```python
from build123d import *

# Parameters (mm, degrees)
F0_R     = 6
F1_DEPTH = 25
F3_DEPTH = 12.5


with BuildPart() as f1:
    # F0 (on Front) → F1 (new body)
    with BuildSketch(Plane.XZ):
        with BuildLine():
            ThreePointArc((-34.439272, -8.041347), (-32.264663, -4.27924), (-31.509368, 0))
            ThreePointArc((-31.509368, 0), (-32.24635, 4.228641), (-34.370393, 7.958653))
            ThreePointArc((-34.370393, 7.958653), (-56.509252, 0.053811), (-34.439272, -8.041347))
        make_face()
        with Locations((-44.009368, 0)):
            Circle(F0_R, mode=Mode.SUBTRACT)
        with BuildLine():
            ThreePointArc((-34.370393, 7.958653), (-32.24635, 4.228641), (-31.509368, 0))
            ThreePointArc((-31.509368, 0), (-32.264663, -4.27924), (-34.439272, -8.041347))
            Line((-34.439272, -8.041347), (35.046161, -8.041347))
            ThreePointArc((35.046161, -8.041347), (30.99087, -0.068914), (34.935895, 7.958653))
            Line((34.935895, 7.958653), (-34.370393, 7.958653))
        make_face()
        with BuildLine():
            ThreePointArc((50.990632, 0), (45.432064, 8.959558), (34.935895, 7.958653))
            ThreePointArc((34.935895, 7.958653), (30.99087, -0.068914), (35.046161, -8.041347))
            ThreePointArc((35.046161, -8.041347), (45.493703, -8.928738), (50.990632, 0))
        make_face()
        with Locations((40.990632, 0)):
            Circle(F0_R, mode=Mode.SUBTRACT)
    extrude(amount=F1_DEPTH)

    # F2 (on Top) → F3 (intersect, symmetric)
    with BuildSketch(Plane.XY):
        Polygon((-27.554982, -9), (-56.499865, -9), (-56.499865, -18), (-26.767584, -18), (24.273953, -9), (51.126346, -9), (51.126346, 0), (23.486555, 0), align=None)
    extrude(amount=F3_DEPTH, both=True, mode=Mode.INTERSECT)


solid = f1.part
```
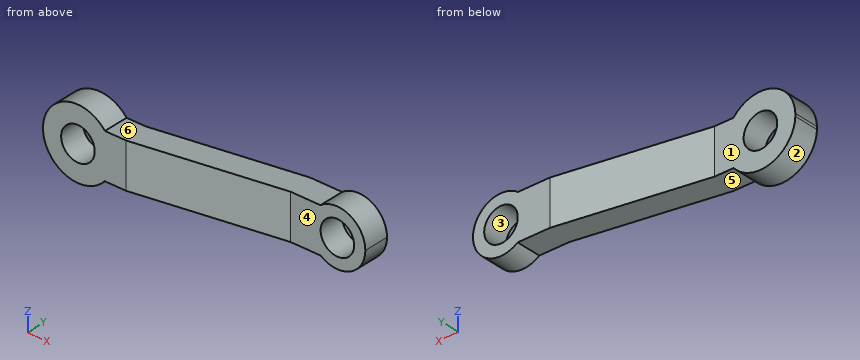
Can you work these out from the model? Positions are in its coordinate system, mm. Face numbers are marked on the shaded views. A direction names the side the tool comes from. Give positions to 0.01 mm unless a question says otherwise; leave off trailing zeros. Loops run counter-clockwise (first coordinate to the right, second up) from the corner with the lowest first, then second, coordinate; pieces in that order, holes last. Notation, with made-up numbers: M -28,-35 L -18,-35 A21 ccw -18,-9 Z; hole C -31.75,39.25 d3. An arc over 180 degrees is marked long. One line per item, written item: value.
(1) Will these pins go through, and if not, where does the flat tip stop? pin 1 (3 mm diameter, centred on x = -19.5, z = -6, fed in from +Y); pin 2 (6 mm diameter, centred on x = 38, z = -2, fed in from -Y); pin 3 (5.5 mm diameter, centred on x = 5, y = -9.5, fed in from -Z).
Returned:
pin 1: y = -7.32
pin 2: y = -9
pin 3: z = -8.04
(2) I need wall thicknesses on line 1 (Y direction, x = 28.5, z = -2.75); line 2 (Z direction, x = -19.5, y = -9.75); line 3 (Y direction, x = -35, z = -7). Which ranges of each line are inside material? Lowest first, please.
Returned:
line 1: -9 to 0
line 2: -8.04 to 7.96
line 3: -18 to -9
(3) Suppose I cut it at D-D on y = -4.5. List the corners of the cut face in (x, z) for me.
Returned:
outline: M -2.03,-8.04 L 35.05,-8.04 A10 ccw long 34.94,7.96 L -2.03,7.96 Z; hole C 40.99,0 d12
(4) We'd pull the mould along Z, two halves only. Please class the marked faces 1, 2 and 3: released by +Z, released by -Z, zero draft, split by the parting line, or undercut.
Returned:
face 1: zero draft
face 2: released by -Z
face 3: undercut
(5) Suppose I cut it at B-B on y = -11. List the corners of the cut face in (x, z) for me.
Returned:
outline: M -56.5,-0.49 A12.5 ccw -34.44,-8.04 L 12.93,-8.04 L 12.93,7.96 L -34.37,7.96 A12.5 ccw -56.5,0.49 Z; hole C -44.01,0 d12
(6) Suppose I cut it at A-A on z = 3. List the corners of the cut face in (x, y) for me.
Returned:
outline: M -56.14,-18 L -49.21,-18 L -49.21,-9 L -56.14,-9 Z; M -38.81,-18 L -26.77,-18 L 24.27,-9 L 35.79,-9 L 35.79,0 L 23.49,0 L -27.55,-9 L -38.81,-9 Z; M 46.19,-9 L 50.53,-9 L 50.53,0 L 46.19,0 Z
(7) Suppose I cut it at C-C on x = 36.5. List the corners of the cut face in (y, z) for me (3 decimals), plus the area to 3 significant figures.
Returned:
outline: M -9,-8.935 L 0,-8.935 L 0,-3.979 L -9,-3.979 Z; M -9,3.979 L 0,3.979 L 0,8.935 L -9,8.935 Z
area: 89.2 mm^2
(8) Which directions (+Z, -Z, +X, -X, +Y, -Y) give clear straight access to the entire face, cutting with the end or side of a thin tool? Please do the marked faces 4, 5 and 6.
Returned:
face 4: +Z, -Z, +X, -Y
face 5: -Z, +Y, -Y
face 6: +Z, +Y, -Y
